```python
from build123d import *

# Parameters (mm, degrees)
ESQUISSE1_R                   = 175
BOSS_EXTRU_1_DEPTH            = 5
ESQUISSE2_R                   = 4.7
ENL_V_MAT_EXTRU_1_DEPTH       = 5
LEDS_BOUT_TIRETTE_R           = 10.7
LEDS_BOUT_TIRETTE_R_2         = 4
LEDS_BOUT_TIRETTE_R_3         = 5
LEDS_BOUT_TIRETTE_W           = 30
LEDS_BOUT_TIRETTE_H           = 11
LEDS_BUTTONS_DEPTH            = 10
FIXATION_ACENSSEURS_R         = 1.5
ENL_V_MAT_EXTRU_2_DEPTH       = 10
ENL_V_MAT_EXTRU_3_DEPTH       = 10
ENL_V_MAT_EXTRU_4_DEPTH       = 10
ENL_V_START                   = -2.417292656
ENL_V_MAT_EXTRU_5_OUTLINE_W   = 7.070312755
ENL_V_MAT_EXTRU_5_OUTLINE_H   = 5
ENL_V_MAT_EXTRU_5_DEPTH       = 20
ENL_V_START_2                 = -32.417292656
ENL_V_MAT_EXTRU_5_2_OUTLINE_W = 10
ENL_V_MAT_EXTRU_5_2_OUTLINE_H = 5
ENL_V_MAT_EXTRU_5_2_DEPTH     = 5
ENL_V_START_3                 = 42.582707344
ENL_V_MAT_EXTRU_5_3_OUTLINE_W = 10
ENL_V_MAT_EXTRU_5_3_OUTLINE_H = 5
ENL_V_MAT_EXTRU_5_3_DEPTH     = 5
ENL_V_START_4                 = -27.417292656
ENL_V_MAT_EXTRU_5_4_OUTLINE_W = 7.070312755
ENL_V_MAT_EXTRU_5_4_OUTLINE_H = 5
ENL_V_MAT_EXTRU_5_4_DEPTH     = 5
ENL_V_START_5                 = 37.582707344
ENL_V_MAT_EXTRU_5_5_OUTLINE_W = 7.070312755
ENL_V_MAT_EXTRU_5_5_OUTLINE_H = 5
ENL_V_MAT_EXTRU_5_5_DEPTH     = 5
ESQUISSE8_W                   = 10
ESQUISSE8_H                   = 5
ENL_V_MAT_EXTRU_6_DEPTH       = 5
ENL_V_MAT_EXTRU_7_DEPTH       = 10
TROU_TARAUD_M51_D             = 4.2


# Read off the part's stored shape, not the designer's step: Enlèv. mat.-Extru.5
with BuildPart() as part:
    # Esquisse1 → Boss.-Extru.1 (new body)
    with BuildSketch(Plane.XY):
        Circle(ESQUISSE1_R)
    extrude(amount=BOSS_EXTRU_1_DEPTH)

    # Esquisse2 → Enlèv. mat.-Extru.1 (cut)
    with BuildSketch(Plane(origin=(0, 0, 0), x_dir=(-1, 0, 0), z_dir=(0, 0, -1))):
        with Locations((-18.220426897, 85.887612711)):
            Circle(ESQUISSE2_R)
        with Locations((40.460378836, 115.887612711)):
            Circle(ESQUISSE2_R)
        with Locations((-65.270641029, -58.723158916)):
            Circle(ESQUISSE2_R)
        with Locations((-120.59180601, -22.904090436)):
            Circle(ESQUISSE2_R)
        Polygon((26.7795731, 95.88761271), (38.263317053, 161.015161015), (68.550112498, 161.015161015), (68.550112498, 190.246123658), (-94.990966298, 190.246123658), (-94.990966298, 161.015161015), (-64.704170853, 161.015161015), (-53.2204269, 95.88761271), align=None)
        Polygon((-96.430895065, -24.752015748), (-158.57487836, -47.370575906), (-173.718276082, -21.141441652), (-199.033032308, -35.756922974), (-117.262492911, -177.387651773), (-91.947736684, -162.772170451), (-107.091134406, -136.543036197), (-56.430895065, -94.034048051), align=None)
    extrude(amount=-ENL_V_MAT_EXTRU_1_DEPTH, mode=Mode.SUBTRACT)

    # Leds, bout., tirette → Leds, buttons (cut)
    with BuildSketch(Plane.XY.offset(5)):
        with Locations((-105, 0)):
            Circle(LEDS_BOUT_TIRETTE_R)
        with Locations((-140, 30)):
            Circle(LEDS_BOUT_TIRETTE_R_2)
        with Locations((-140, -30)):
            Circle(LEDS_BOUT_TIRETTE_R_2)
        with Locations((-160, 15)):
            Circle(LEDS_BOUT_TIRETTE_R_2)
        with Locations((-160, -15)):
            Circle(LEDS_BOUT_TIRETTE_R_3)
        with BuildLine():
            Line((-140, -4.6), (-147.25, -4.6))
            Line((-147.25, -4.6), (-147.25, 4.6))
            Line((-147.25, 4.6), (-140, 4.6))
            ThreePointArc((-140, 4.6), (-135.4, 0), (-140, -4.6))
        make_face()
        with Locations((-110, 30)):
            Rectangle(LEDS_BOUT_TIRETTE_W, LEDS_BOUT_TIRETTE_H)
        with Locations((-110, -30)):
            Rectangle(LEDS_BOUT_TIRETTE_W, LEDS_BOUT_TIRETTE_H)
    extrude(amount=-LEDS_BUTTONS_DEPTH, mode=Mode.SUBTRACT)

    # Fixation acensseurs → Enlèv. mat.-Extru.2 (cut)
    with BuildSketch(Plane(origin=(0, 0, 0), x_dir=(-1, 0, 0), z_dir=(0, 0, -1))):
        with Locations((38.72389706, 106.03953518)):
            Circle(FIXATION_ACENSSEURS_R)
        with Locations((-28.220426897, 85.887612711)):
            Circle(FIXATION_ACENSSEURS_R)
        with Locations((44.280638745, 137.553383277)):
            Circle(FIXATION_ACENSSEURS_R)
        with Locations((3.779573103, 85.887612711)):
            Circle(FIXATION_ACENSSEURS_R)
        with Locations((-111.194879802, -19.483889003)):
            Circle(FIXATION_ACENSSEURS_R)
        with Locations((-60.270641029, -67.383412953)):
            Circle(FIXATION_ACENSSEURS_R)
        with Locations((-141.265043667, -30.428533589)):
            Circle(FIXATION_ACENSSEURS_R)
        with Locations((-76.270641029, -39.670600032)):
            Circle(FIXATION_ACENSSEURS_R)
    extrude(amount=-ENL_V_MAT_EXTRU_2_DEPTH, mode=Mode.SUBTRACT)

    # Esquisse3 → Enlèv. mat.-Extru.3 (cut)
    with BuildSketch(Plane(origin=(0, 0, 0), x_dir=(-1, 0, 0), z_dir=(0, 0, -1))):
        with BuildLine():
            Line((22.704747883, -39.988138527), (44.77437947, -19.667425901))
            Line((44.77437947, -19.667425901), (31.982809207, -5.77493855))
            ThreePointArc((31.982809207, -5.77493855), (-25.570164707, 20.060325942), (13.221748658, -29.68897712))
            Line((13.221748658, -29.68897712), (22.704747883, -39.988138527))
        make_face()
    extrude(amount=-ENL_V_MAT_EXTRU_3_DEPTH, mode=Mode.SUBTRACT)

    # Esquisse4 → Enlèv. mat.-Extru.4 (cut)
    with BuildSketch(Plane(origin=(0, 0, -5), x_dir=(-1, 0, 0), z_dir=(0, 0, -1))):
        Polygon((134.678427666, -65.79510224), (143.338681704, -70.79510224), (140.838681704, -75.125229259), (132.178427666, -70.125229259), align=None)
        Polygon((101.867538534, -52.625229259), (110.527792572, -57.625229259), (113.027792572, -53.29510224), (104.367538534, -48.29510224), align=None)
        Polygon((104.367538534, 48.29510224), (101.867538534, 52.625229259), (110.527792572, 57.625229259), (113.027792572, 53.29510224), align=None)
        Polygon((132.178427666, 70.125229259), (134.678427666, 65.79510224), (143.338681704, 70.79510224), (140.838681704, 75.125229259), align=None)
    extrude(amount=-ENL_V_MAT_EXTRU_4_DEPTH, mode=Mode.SUBTRACT)

    # Enlèv. mat.-Extru.5 outline → Enlèv. mat.-Extru.5 (cut)
    with BuildSketch(Plane(origin=(0, 0, 0), x_dir=(0.899482426544107, 0.4369569364803871, 0), z_dir=(0.4369569364803871, -0.8994824265441071, 0)).offset(ENL_V_START)):
        with Locations((162.91185011, 2.5)):
            Rectangle(ENL_V_MAT_EXTRU_5_OUTLINE_W, ENL_V_MAT_EXTRU_5_OUTLINE_H)
    extrude(amount=ENL_V_MAT_EXTRU_5_DEPTH, mode=Mode.SUBTRACT)

    # Enl_v. mat.-Extru.5 2 outline → Enl_v. mat.-Extru.5 2 (cut)
    with BuildSketch(Plane(origin=(0, 0, 0), x_dir=(0.899482426544107, 0.4369569364803871, 0), z_dir=(0.4369569364803871, -0.8994824265441071, 0)).offset(ENL_V_START_2)):
        with Locations((117.627599257, 2.5)):
            Rectangle(ENL_V_MAT_EXTRU_5_2_OUTLINE_W, ENL_V_MAT_EXTRU_5_2_OUTLINE_H)
        with Locations((151.447761545, 2.5)):
            Rectangle(ENL_V_MAT_EXTRU_5_2_OUTLINE_W, ENL_V_MAT_EXTRU_5_2_OUTLINE_H)
    extrude(amount=ENL_V_MAT_EXTRU_5_2_DEPTH, mode=Mode.SUBTRACT)

    # Enl_v. mat.-Extru.5 3 outline → Enl_v. mat.-Extru.5 3 (cut)
    with BuildSketch(Plane(origin=(0, 0, 0), x_dir=(0.899482426544107, 0.4369569364803871, 0), z_dir=(0.4369569364803871, -0.8994824265441071, 0)).offset(ENL_V_START_3)):
        with Locations((117.627599257, 2.5)):
            Rectangle(ENL_V_MAT_EXTRU_5_3_OUTLINE_W, ENL_V_MAT_EXTRU_5_3_OUTLINE_H)
        with Locations((151.447761545, 2.5)):
            Rectangle(ENL_V_MAT_EXTRU_5_3_OUTLINE_W, ENL_V_MAT_EXTRU_5_3_OUTLINE_H)
    extrude(amount=ENL_V_MAT_EXTRU_5_3_DEPTH, mode=Mode.SUBTRACT)

    # Enl_v. mat.-Extru.5 4 outline → Enl_v. mat.-Extru.5 4 (cut)
    with BuildSketch(Plane(origin=(0, 0, 0), x_dir=(0.899482426544107, 0.4369569364803871, 0), z_dir=(0.4369569364803871, -0.8994824265441071, 0)).offset(ENL_V_START_4)):
        with Locations((162.91185011, 2.5)):
            Rectangle(ENL_V_MAT_EXTRU_5_4_OUTLINE_W, ENL_V_MAT_EXTRU_5_4_OUTLINE_H)
    extrude(amount=ENL_V_MAT_EXTRU_5_4_DEPTH, mode=Mode.SUBTRACT)

    # Enl_v. mat.-Extru.5 5 outline → Enl_v. mat.-Extru.5 5 (cut)
    with BuildSketch(Plane(origin=(0, 0, 0), x_dir=(0.899482426544107, 0.4369569364803871, 0), z_dir=(0.4369569364803871, -0.8994824265441071, 0)).offset(ENL_V_START_5)):
        with Locations((162.91185011, 2.5)):
            Rectangle(ENL_V_MAT_EXTRU_5_5_OUTLINE_W, ENL_V_MAT_EXTRU_5_5_OUTLINE_H)
    extrude(amount=ENL_V_MAT_EXTRU_5_5_DEPTH, mode=Mode.SUBTRACT)

    # Esquisse8 → Enlèv. mat.-Extru.6 (cut)
    with BuildSketch(Plane(origin=(0, 0, 0), x_dir=(-1, 0, 0), z_dir=(0, 0, -1))):
        with Locations((53.5, 60.88761271)):
            Rectangle(ESQUISSE8_W, ESQUISSE8_H)
        with Locations((5, 60.88761271)):
            Rectangle(ESQUISSE8_W, ESQUISSE8_H)
        with Locations((-43.5, 60.88761271)):
            Rectangle(ESQUISSE8_W, ESQUISSE8_H)
        Polygon((-79.145282892, 10.308425729), (-74.145282892, 1.648171691), (-69.815155873, 4.148171691), (-74.815155873, 12.808425729), align=None)
        Polygon((-54.895282892, -31.693806355), (-49.895282892, -40.354060393), (-45.565155873, -37.854060393), (-50.565155873, -29.193806355), align=None)
        Polygon((-21.315155873, -79.856292476), (-26.315155873, -71.196038439), (-30.645282892, -73.696038439), (-25.645282892, -82.356292476), align=None)
    extrude(amount=-ENL_V_MAT_EXTRU_6_DEPTH, mode=Mode.SUBTRACT)

    # Esquisse9 → Enlèv. mat.-Extru.7 (cut)
    with BuildSketch(Plane(origin=(0, 0, 0), x_dir=(-1, 0, 0), z_dir=(0, 0, -1))):
        with BuildLine():
            Line((143.351607751, -100.375876361), (89.833936865, -62.90239978))
            ThreePointArc((89.833936865, -62.90239978), (22.830586532, -107.264217842), (-56.430895065, -94.034048051))
            Line((-56.430895065, -94.034048051), (-107.091134406, -136.543036197))
            Line((-107.091134406, -136.543036197), (-105.168163584, -139.873719363))
            ThreePointArc((-105.168163584, -139.873719363), (38.840643584, -244.384683529), (143.351607751, -100.375876361))
        make_face()
    extrude(amount=-ENL_V_MAT_EXTRU_7_DEPTH, mode=Mode.SUBTRACT)

    # Trou taraudé M51 (through all)
    with Locations(Plane(origin=(0, 0, -5), x_dir=(1, 0, 0), z_dir=(0, 0, -1))):
        with Locations((-68.568956805, -27.662548456), (55.280905682, -37.98337033), (-87.299337242, 135.559338217)):
            Hole(TROU_TARAUD_M51_D / 2)


solid = part.part
```
CAD build for the part. Positions are in the model's coordinates, mm. A direction names the side the tool comes from. Coordinates: 2 decimals unless noted, no trailing zeros. Order: outer loops, then holes, each group sorted by start corner. A loop starts at its lowest first (then second) coordinate and runs counter-clockwise, first axis right, second up. Notation, with made-up numbers: M 83.25,48 L 126.25,48 A28 ccw 126.25,67 Z; hole C -6.5,16.25 d11. An arc over 180 degrees is marked long. Write each question's results on one line, items separated by ' | '. Start each with the question number.
Q1. Cut at B-B (z = 4). Count the separate pieces of the cut face and the enclosed holes in it, then the cut area to 3 significant figures.
Q2. Which spindle directions (+Z, -Z, +X, -X, +Y, -Y) get a long thin tool onto all of the face, cutting with end or side? Do faces 1 (the flat face through (76.15, -59.88, 2.46)), 2 (the flat face through (59.043, 128.907, 2.465)), 3 (the flat face through (152.968, 66.036, 2.465)), 4 (the cylindrical face through (-167.634, 50.238, 2.465)). Say none if no direction does.
Q3. Cut at A-A (x = -160). List the corners of the cut face in (y, z), then the cut area to 3 significant figures.
Q4. Drill centre lines: probe 1 along X at (y, z) = (67, 1.25); probe 2 along X at (y, z) = (58.5, 0.6); probe 3 along Y at (x, z) = (2, 0.8). Where is each one in solid material? Low to high. Write a range as from..to.
Q5. Flat gauge pins, fed straight in: P1, Ø4, axis at x = 55.28, y = 37.98, coming from the -Z side; P2, Ø3, axis at x = 79, z = 2, coming from the +Y side; P3, Ø1.5, axis at y = 91, z = 3.5, coming from the +X side; P4, Ø1.5, axis at y = 78, z = 2, coming from the -X side. Where does each tip first touch, or does it go through?
Q6. Pull direction Y, two halves, no side cores. Call faces 5 (the flat face through (-41, 28, 0)), 6 (the cylindrical face through (19.24, 81.3, 2.46)), 7 (the flat face through (166.04, -34.44, 2.46)): +Y half, -Y half, draft (parallel to the pull), parting line (faces both ways), or undercut.
Found:
1) separate pieces: 1 | enclosed holes: 40 | area: 60,700 mm²
2) face 1: +Z, -Z, -Y | face 2: +Z, -Z, +Y | face 3: +Z, -Z | face 4: +Z, -Z, -X
3) outline: M -70.89,0 L -20,0 L -20,5 L -70.89,5 Z; M -10,0 L 11,0 L 11,5 L -10,5 Z; M 19,0 L 70.89,0 L 70.89,5 L 19,5 Z | area: 619 mm²
4) probe 1: -161.67..-136.77, -133.98..144.64, 152.5..161.67 | probe 2: -164.93..-58.5, -48.5..-10, 0..38.5, 48.5..148.77, 156.63..164.93 | probe 3: -109.65..-32.44, 32.44..95.89
5) P1: through | P2: y = 156.9 | P3: x = 149.93 | P4: x = -157.03
6) face 5: draft | face 6: undercut | face 7: -Y half
